Design review of the part built by this model. Coordinates are the model's own, in mm. A direction names the side the tool comes from. Round coordinates to 2 decimals unless told otherwise and drop trailing zeros. Loops run counter-clockwise (first coordinate to the right, second up) from the corner with the lowest first, then second, coordinate; pieces in that order, holes last. Notation, with made-up numbers: M -27.75,28.25 L 16.25,28.25 A34 ccw 16.25,58.25 Z; hole C 82.5,-7.5 d10. An arc over 180 degrees is marked long. One line per item, written item: value. Start each with the question number.
Item 1: Clearance check with flat-ended pins moving along their axes: pin 1 (15 mm diameter, centred on y = 58.5, z = 33, fed in from -X); pin 2 (8 mm diameter, centred on x = 30.5, z = -884.5, fed in from +Y); pin 3 (10 mm diameter, centred on x = 54.5, y = 22, fed in from +Z). State where each tip first meets the part, or that it passes through.
Item 2: For line 1 along Z through (x, y) = (-20, 103.5); line 2 along Z through (x, y) = (79, -152); line 3 along Z through (x, y) = (-26.5, -214.5), list the stretches that pass through material, from the lowest coordinate up.
Item 3: We need section A-A (y = -207.5). State how many separate pieces and enclosed holes the cut face has, then the cut area to 3 significant figures.
Item 4: Mouldability with a two-part tool opening along Z and no side actions: class faces 1 (the flat face through (2, 71, -550)), 2 (the cylindrical face through (-87.832, -61.468, 24.65)), 3 (the flat face through (-1, -29, 250)) as released by +Z, released by -Z, zero draft, split by the parting line, or undercut.
Item 5: We need section C-C (z = -626). Write out the cut boundary in (x, y).
Item 6: We need section B-B (x = -105.5). Write out the cut boundary in (y, z), then the cut area to 3 significant figures.
Item 7: For faces 4 (the flat face through (1.05, -179.486, -561.877)), 5 (the flat face through (75, 44, -1025)), 6 (the cylindrical face through (-1.65, -104.98, -865.04)), list the 3-axis set-ups (+Z, -Z, +X, -X, +Y, -Y) from which the entire face can be reached by the end or side of a thin tool; tool diameter is ignored.
from build123d import *

# Parameters (mm, degrees)
BOSS_EXTRUDE1_DEPTH  = 50
CUT_EXTRUDE1_DEPTH   = 246
SKETCH6_R            = 70
BOSS_EXTRUDE2_DEPTH  = 100
BOSS_EXTRUDE3_DEPTH  = 50
SKETCH8_R            = 70
BOSS_EXTRUDE4_DEPTH  = 100
BOSS_EXTRUDE5_DEPTH  = 50
SKETCH10_R           = 70
BOSS_EXTRUDE6_DEPTH  = 100
BOSS_EXTRUDE7_DEPTH  = 50
SKETCH12_R           = 70
BOSS_EXTRUDE8_DEPTH  = 50
SKETCH13_R           = 70
BOSS_EXTRUDE9_DEPTH  = 50
SKETCH14_R           = 50
BOSS_EXTRUDE11_DEPTH = 150
CUT_EXTRUDE2_DEPTH   = 246


with BuildPart() as part:
    # Sketch1 → Boss-Extrude1 (new body)
    with BuildSketch(Plane.XY):
        with BuildLine():
            Line((-75, 120), (-75, -30))
            ThreePointArc((-75, -30), (-88.180194847, -61.819805153), (-120, -75))
            ThreePointArc((-120, -75), (-161.602514717, -97.264990189), (-166.153846154, -144.230769231))
            ThreePointArc((-166.153846154, -144.230769231), (0, -255), (166.153846154, -144.230769231))
            ThreePointArc((166.153846154, -144.230769231), (161.602514717, -97.264990189), (120, -75))
            ThreePointArc((120, -75), (88.180194847, -61.819805153), (75, -30))
            Line((75, -30), (75, 120))
            ThreePointArc((75, 120), (0, 195), (-75, 120))
        make_face()
    extrude(amount=BOSS_EXTRUDE1_DEPTH)

    # Sketch5 → Cut-Extrude1 (cut, through all)
    with BuildSketch(Plane(origin=(75, 0, 0), x_dir=(0, 0, -1), z_dir=(1, 0, 0))):
        Polygon((-50, 70), (-50, 195), (-20, 195), align=None)
    extrude(amount=-CUT_EXTRUDE1_DEPTH, mode=Mode.SUBTRACT)

    # Sketch6 → Boss-Extrude2 (add)
    with BuildSketch(Plane(origin=(0, 0, 0), x_dir=(-1, 0, 0), z_dir=(0, 0, -1))):
        with Locations((0, 120)):
            Circle(SKETCH6_R)
    extrude(amount=BOSS_EXTRUDE2_DEPTH)

    # Sketch7 → Boss-Extrude3 (add)
    with BuildSketch(Plane(origin=(0, 0, -100), x_dir=(-1, 0, 0), z_dir=(0, 0, -1))):
        with BuildLine():
            Line((75, 120), (75, -30))
            ThreePointArc((75, -30), (0, -105), (-75, -30))
            Line((-75, -30), (-75, 120))
            ThreePointArc((-75, 120), (0, 195), (75, 120))
        make_face()
    extrude(amount=BOSS_EXTRUDE3_DEPTH)

    # Sketch8 → Boss-Extrude4 (add)
    with BuildSketch(Plane(origin=(0, 0, -150), x_dir=(-1, 0, 0), z_dir=(0, 0, -1))):
        with Locations((0, -30)):
            Circle(SKETCH8_R)
    extrude(amount=BOSS_EXTRUDE4_DEPTH)

    # Sketch9 → Boss-Extrude5 (add)
    with BuildSketch(Plane(origin=(0, 0, -250), x_dir=(-1, 0, 0), z_dir=(0, 0, -1))):
        with BuildLine():
            Line((75, -30), (75, -180))
            ThreePointArc((75, -180), (0, -255), (-75, -180))
            Line((-75, -180), (-75, -30))
            ThreePointArc((-75, -30), (0, 45), (75, -30))
        make_face()
    extrude(amount=BOSS_EXTRUDE5_DEPTH)

    # Sketch10 → Boss-Extrude6 (add)
    with BuildSketch(Plane(origin=(0, 0, -300), x_dir=(-1, 0, 0), z_dir=(0, 0, -1))):
        with Locations((0, -180)):
            Circle(SKETCH10_R)
    extrude(amount=BOSS_EXTRUDE6_DEPTH)

    # Sketch11 → Boss-Extrude7 (add)
    with BuildSketch(Plane(origin=(0, 0, -400), x_dir=(-1, 0, 0), z_dir=(0, 0, -1))):
        with BuildLine():
            Line((75, -180), (75, -30))
            ThreePointArc((75, -30), (88.180194847, 1.819805153), (120, 15))
            ThreePointArc((120, 15), (161.602514717, 37.264990189), (166.153846154, 84.230769231))
            ThreePointArc((166.153846154, 84.230769231), (0, 195), (-166.153846154, 84.230769231))
            ThreePointArc((-166.153846154, 84.230769231), (-161.602514717, 37.264990189), (-120, 15))
            ThreePointArc((-120, 15), (-88.180194847, 1.819805153), (-75, -30))
            Line((-75, -30), (-75, -180))
            ThreePointArc((-75, -180), (0, -255), (75, -180))
        make_face()
    extrude(amount=BOSS_EXTRUDE7_DEPTH)

    # Sketch12 → Boss-Extrude8 (add)
    with BuildSketch(Plane(origin=(0, 0, -450), x_dir=(-1, 0, 0), z_dir=(0, 0, -1))):
        with Locations((0, -30)):
            Circle(SKETCH12_R)
    extrude(amount=BOSS_EXTRUDE8_DEPTH)

    # Sketch13 → Boss-Extrude9 (add)
    with BuildSketch(Plane.XY.offset(50)):
        with Locations((0, -30)):
            Circle(SKETCH13_R)
    extrude(amount=BOSS_EXTRUDE9_DEPTH)

    # Sketch14 → Boss-Extrude11 (add)
    with BuildSketch(Plane.XY.offset(100)):
        with Locations((0, -30)):
            Circle(SKETCH14_R)
    extrude(amount=BOSS_EXTRUDE11_DEPTH)

    # Sketch15 → Cut-Extrude2 (cut, through all)
    with BuildSketch(Plane(origin=(75, 0, 0), x_dir=(0, 0, -1), z_dir=(1, 0, 0))):
        Polygon((100, 20), (100, -105), (130, -105), align=None)
        Polygon((150, 70), (150, 195), (120, 195), align=None)
        Polygon((300, -80), (300, 45), (270, 45), align=None)
        Polygon((250, -130), (250, -255), (280, -255), align=None)
        Polygon((450, -130), (450, -255), (420, -255), align=None)
    extrude(amount=-CUT_EXTRUDE2_DEPTH, mode=Mode.SUBTRACT)

    # Mirror2: part across plane


with BuildPart() as part_1:
    add(part.part)
    add(part.part.mirror(Plane(origin=(0, -30, -500), x_dir=(1, 0, 0), z_dir=(0, 0, -1))))


solid = part_1.part
A:
1. pin 1: x = -75
1. pin 2: y = 190.16
1. pin 3: z = 50
2. line 1: -1041.96 to -858.04, -600 to -550, -450 to -400, -141.96 to 41.96
2. line 2: -1050 to -1000, 0 to 50
2. line 3: -1050 to -1000, -729.72 to -570.28, -429.72 to -270.28, 0 to 50
3. separate pieces: 4
3. enclosed holes: 0
3. area: 67,600 mm2
4. face 1: undercut
4. face 2: zero draft
4. face 3: released by +Z
5. outline: C 0,-180 d140
6. outline: M -220.84,-1050 L -72.6,-1050 L -72.6,-1000 L -220.84,-1000 Z; M -220.84,0 L -72.6,0 L -72.6,50 L -220.84,50 Z; M 12.6,-600 L 160.84,-600 L 160.84,-550 L 12.6,-550 Z; M 12.6,-450 L 160.84,-450 L 160.84,-400 L 12.6,-400 Z
6. area: 29,600 mm2
7. face 4: +X, -X, -Y
7. face 5: -Z, +X, +Y
7. face 6: -Y
